Geometry: final body of the model. Coordinates: model frame, mm. A direction names the side the tool comes from. Give positions to 0.01 mm unless a question says otherwise; leave off trailing zeros. Write each loop counter-clockwise with the first axis right and the second up, starting at its lowest first coordinate (ties: lowest second). Pieces come first, ordered by that corner, then holes. Notation, with made-up numbers: (29.5, 82.5) -> (43.5, 82.5) arc R26 ccw to (43.5, 108.5) -> close; hole circle Ø10 at (48, 14). An arc over 180 degrees is marked (long way). Answer as a JSON object with one key per item and string values. Group by question number.
(1) Section query B-B on y = 14.25. Output: boundary loops of the cut face in (x, z), plus the area to 3 significant figures.
(2) Section query A-A on x = 17.5. Output: boundary loops of the cut face in (y, z).
(3) Material intervals for probe 1 along X at (y, z) = (10.25, 0); probe 2 along Z at (x, y) = (0, 13.5); probe 3 along X at (y, z) = (11.25, 0.5), sorted ascending.
(4) Contact query for flat-ended pins moving along their axis: pin 1 Ø1 at (x, z) = (17, 3) entering from +Y; pin 2 Ø2 at (x, y) = (14.5, 1) entering from -Z; pin 3 Ø3 at (y, z) = (11.5, 3) entering from +X. Output: stop coordinate, or through.
(5) Draft query along Z for faces 1 (the face through (25.13, 5.83, -0.02)), 2 (the face through (2.793, 1.237, 3.112)), 3 (the face through (12, 1, -3)). Return one class per face: +Z half, -Z half, draft (parallel to the pull), parting line (faces both ways), or undercut.
(6) Set-up query: faces 4 (the face through (25.732, 11.13, -0.163)), 5 (the face through (2.815, 1.237, -3.106)), 6 (the face through (22.185, 1.237, 3.106)). Return all of +Z, -Z, +X, -X, +Y, -Y with unobstructed straight access to the full face (end or side cutting, diameter ignored); none if empty.
Autodesk Inventor part; units mm, degrees
ref_plane "YZ Plane" through (0, 0, 0) normal (1, 0, 0) x (0, 1, 0)
ref_plane "XZ Plane" through (0, 0, 0) normal (0, 1, 0) x (-1, 0, 0)
ref_plane "XY Plane" through (0, 0, 0) normal (0, 0, 1) x (1, 0, 0)
sketch "Esboço1" plane through (0, 0, 0) normal (0, 1, 0) x (-1, 0, 0)
  arc A0 (-2.0603, -3.4286) -> (-2.0603, 3.4286) centre (0, 0) ccw
  arc A1 (-22.9397, 3.4286) -> (-22.9397, -3.4286) centre (-25, 0) ccw
  line L0 (-3.6056, -3) -> (-21.3944, -3)
  line L1 (-3.6056, 3) -> (-21.3944, 3)
  arc A2 (-2.0603, -3.4286) -> (-3.6056, -3) centre (-3.6056, -6) ccw
  arc A3 (-3.6056, 3) -> (-2.0603, 3.4286) centre (-3.6056, 6) ccw
  arc A4 (-21.3944, -3) -> (-22.9397, -3.4286) centre (-21.3944, -6) ccw
  arc A5 (-22.9397, 3.4286) -> (-21.3944, 3) centre (-21.3944, 6) ccw
  point P0 (-2.6458, -3)
  point P1 (-22.3542, -3)
  point P2 (-2.6458, 3)
  point P3 (-22.3542, 3)
  dimension "d3" = 6
  dimension "d5" = 3
  dimension "d11" = 25
  dimension "d13" = 4
extrude "Extrusão1" add sketch "Esboço1" along normal blind 2.5
fillet "Arredondamento1" radius 0.3 16 edges at (22.1962, 0, 3.1091) (29, 0, 0) (22.1962, 0, -3.1091) (12.5, 0, -3) (2.8038, 0, -3.1091) (-4, 0, 0) (2.8038, 0, 3.1091) (12.5, 0, 3) (22.1962, 2.5, 3.1091) (29, 2.5, 0) (22.1962, 2.5, -3.1091) (12.5, 2.5, -3) (2.8038, 2.5, -3.1091) (-4, 2.5, 0) (2.8038, 2.5, 3.1091) (12.5, 2.5, 3)
sketch "Esboço2" plane through (0, 2.5, 0) normal (0, 1, 0) x (1, 0, 0)
  circle A0 centre (0, 0) radius 2.4
  circle A1 centre (25, 0) radius 2.4
  arc A2 (23.0942, -3.1714) -> (23.0942, 3.1714) centre (25, 0) ccw
  dimension "d14" = 4.8
extrude "Extrusão2" add sketch "Esboço2" along normal blind 13.7
sketch "Esboço3" plane through (0, 16.2, 0) normal (0, 1, 0) x (1, 0, 0)
  circle A0 centre (0, 0) radius 2.4
  circle A1 centre (25, 0) radius 2.4
hole "Furo1" at (0, 16.2, 0) at (25, 16.2, 0) direction (0, -1, 0) diameter 1.5 depth 10 tip angle 118
properties part number "_3DPrint"
Answer list:
{
 "1": {"outline": "circle Ø4.8 at (0, 0); circle Ø4.8 at (25, 0); hole circle Ø1.5 at (0, 0); hole circle Ø1.5 at (25, 0)", "area": "32.7 mm2"},
 "2": {"outline": "(0, -2.7) arc R0.3 ccw to (0.3, -3) -> (2.2, -3) arc R0.3 ccw to (2.5, -2.7) -> (2.5, 2.7) arc R0.3 ccw to (2.2, 3) -> (0.3, 3) arc R0.3 ccw to (0, 2.7) -> close"},
 "3": {"probe 1": "-2.4 to -0.75, 0.75 to 2.4, 22.6 to 24.25, 25.75 to 27.4", "probe 2": "-2.4 to -0.75, 0.75 to 2.4", "probe 3": "-2.35 to -0.56, 0.56 to 2.35, 22.65 to 24.44, 25.56 to 27.35"},
 "4": {"pin 1": "y = 2.5", "pin 2": "z = -3", "pin 3": "x = 26.87"},
 "5": {"face 1": "undercut", "face 2": "+Z half", "face 3": "-Z half"},
 "6": {"face 4": "+Y", "face 5": "-Z, +Y, -Y", "face 6": "+Z, +Y, -Y"}
}
